Can you work these out from the drawing? Everything is in mm from the part's minimum corner. Round coordinates to 2 decimals unless told otherwise and drop trailing zeros. Write each loop counter-clockwise with the first axis right and the second up, starting at its lowest first coordinate (ties: lowest second). Pieces come first, ordered by that corner, then holes. Notation, with made-up numbers: (72, 20.25) - (106, 20.25) arc R22 cw to (106, 48.25) - close; hole circle Ø3 at (54.5, -4). An arc over 180 degrees is marked (long way). One line per item, written item: value. Start each with the question number.
(1) I want a section at B-B on z = 21.25. List the corners of the cut face in (x, y) for me.
(2) I want a section at A-A on y = 0.9. List the corners of the cut face in (x, z) for me, plus the area to 3 significant figures.
(3) I want a section at D-D on x = 82. List the corners of the cut face in (y, z) for me.
(4) I'm going to push flat-ended pins straight in: pin 1 Ø1 at (y, z) = (0.5, 90) entering from -X; pin 2 Ø1 at (x, z) = (65, 77.5) entering from -Y; pin 3 Ø2.5 at (x, z) = (36.25, 21.25) entering from +Y. Where does each tip first touch, or does it pass through?
(5) If I drill on L1, parallel to X at y = 0.8, z = 21.25; L2, parallel to X at y = 1.4, z = 86; L3, parallel to Z at x = 79, y = 0.45, over which ranges is the centre line in solid material (lowest first)? Write a range as from..to.
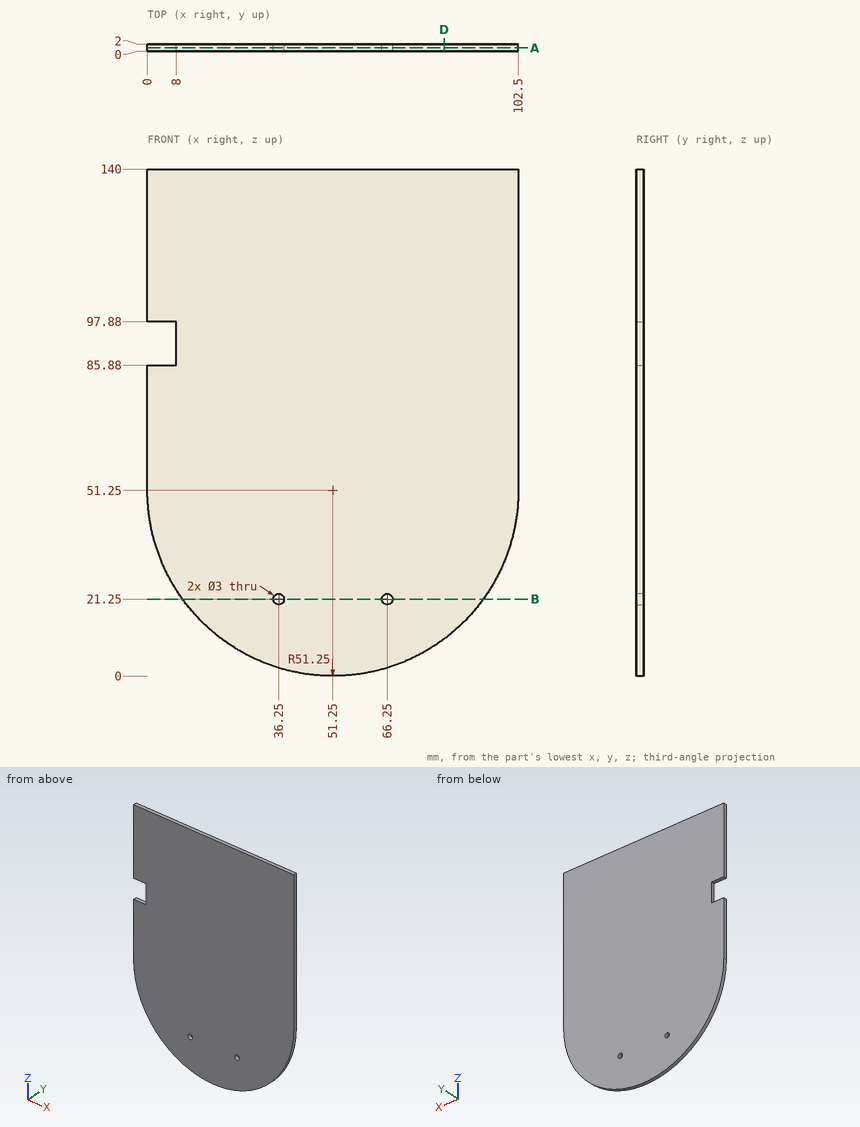
Established:
1. outline: (9.7, 0) - (34.75, 0) - (34.75, 2) - (9.7, 2) - close; (37.75, 0) - (64.75, 0) - (64.75, 2) - (37.75, 2) - close; (67.75, 0) - (92.8, 0) - (92.8, 2) - (67.75, 2) - close
2. outline: (0, 51.25) arc R51.25 ccw to (102.5, 51.25) - (102.5, 140) - (0, 140) - (0, 97.88) - (8, 97.88) - (8, 85.88) - (0, 85.88) - close; hole circle Ø3 at (36.25, 21.25); hole circle Ø3 at (66.25, 21.25)
2. area: 13,100 mm2
3. outline: (0, 10.25) - (2, 10.25) - (2, 140) - (0, 140) - close
4. pin 1: x = 8
4. pin 2: y = 0
4. pin 3: through
5. L1: 9.7..34.75, 37.75..64.75, 67.75..92.8
5. L2: 8..102.5
5. L3: 8.16..140
